from build123d import *

# Parameters (mm, degrees)
CYLINDER009_R     = 5
CYLINDER009_DEPTH = 10
CYLINDER008_R     = 30
CYLINDER008_DEPTH = 10
CYLINDER012_R     = 2
CYLINDER012_DEPTH = 63
CYLINDER013_R     = 2
CYLINDER013_DEPTH = 63
CYLINDER014_R     = 2
CYLINDER014_DEPTH = 63
CYLINDER011_R     = 2
CYLINDER011_DEPTH = 63
BOX004_W          = 86
BOX004_H          = 86
BOX004_DEPTH      = 5
FILLET003_R       = 12
BOX003_W          = 80
BOX003_H          = 80
BOX003_DEPTH      = 1
FILLET002_R       = 12


with BuildPart() as led:
    # Cylinder009 → Cylinder009 (new body)
    with BuildSketch(Plane(origin=(52, 9, -6), x_dir=(1, 0, 0), z_dir=(0, 0, 1))):
        Circle(CYLINDER009_R)
    extrude(amount=CYLINDER009_DEPTH)


with BuildPart() as speaker:
    # Cylinder008 → Cylinder008 (new body)
    with BuildSketch(Plane(origin=(42, 42, -6), x_dir=(1, 0, 0), z_dir=(0, 0, 1))):
        Circle(CYLINDER008_R)
    extrude(amount=CYLINDER008_DEPTH)


with BuildPart() as rod2:
    # Cylinder012 → Cylinder012 (new body)
    with BuildSketch(Plane(origin=(72.6, 72, -9), x_dir=(1, 0, 0), z_dir=(0, 0, 1))):
        Circle(CYLINDER012_R)
    extrude(amount=CYLINDER012_DEPTH)


with BuildPart() as rod3:
    # Cylinder013 → Cylinder013 (new body)
    with BuildSketch(Plane(origin=(12.6, 12, -9), x_dir=(1, 0, 0), z_dir=(0, 0, 1))):
        Circle(CYLINDER013_R)
    extrude(amount=CYLINDER013_DEPTH)


with BuildPart() as rod4:
    # Cylinder014 → Cylinder014 (new body)
    with BuildSketch(Plane(origin=(12.6, 72, -9), x_dir=(1, 0, 0), z_dir=(0, 0, 1))):
        Circle(CYLINDER014_R)
    extrude(amount=CYLINDER014_DEPTH)


with BuildPart() as holes:
    # Cylinder011 → Cylinder011 (new body)
    with BuildSketch(Plane(origin=(72.6, 12, -9), x_dir=(1, 0, 0), z_dir=(0, 0, 1))):
        Circle(CYLINDER011_R)
    extrude(amount=CYLINDER011_DEPTH)

    # Fusion003: union LED, Speaker, rod2, rod3, rod4
    add(led.part)
    add(speaker.part)
    add(rod2.part)
    add(rod3.part)
    add(rod4.part)


with BuildPart() as fillet003:
    # Box004 → Box004 (new body)
    with BuildSketch(Plane.XY):
        with Locations((43, 43)):
            Rectangle(BOX004_W, BOX004_H)
    extrude(amount=BOX004_DEPTH)

    # Fillet003
    fillet003_edges = [fillet003.edges().sort_by_distance(p)[0] for p in [
        (0, 0, 2.5),
        (0, 86, 2.5),
        (86, 0, 2.5),
        (86, 86, 2.5),
    ]]
    fillet(fillet003_edges, radius=FILLET003_R)


with BuildPart() as fillet003_1:
    # Fillet003 placement: moved
    add(fillet003.part.moved(Location((-3, -3, -5))))


with BuildPart() as frontspeaker:
    # Box003 → Box003 (new body)
    with BuildSketch(Plane.XY):
        with Locations((40, 40)):
            Rectangle(BOX003_W, BOX003_H)
    extrude(amount=BOX003_DEPTH)

    # Fillet002
    fillet002_edges = [frontspeaker.edges().sort_by_distance(p)[0] for p in [
        (0, 0, 0.5),
        (0, 80, 0.5),
        (80, 0, 0.5),
        (80, 80, 0.5),
    ]]
    fillet(fillet002_edges, radius=FILLET002_R)

    # Fusion001: union Fillet003
    add(fillet003_1.part)


with BuildPart() as frontspeaker_1:
    # Fusion001 placement: moved
    add(frontspeaker.part.moved(Location((2, 2, 0))))

    # Cut005: cut holes
    add(holes.part, mode=Mode.SUBTRACT)


solid = frontspeaker_1.part
Here's how the part is built. I have some questions about the finished solid (model axes, mm). A direction names the side the tool comes from. Give positions to 0.01 mm unless a question says otherwise; leave off trailing zeros. Order: outer loops, then holes, each group sorted by start corner. A loop starts at its lowest first (then second) coordinate and runs counter-clockwise, first axis right, second up. Notation, with made-up numbers: (41.5, -31) -> (86.5, -31) arc R29 ccw to (86.5, -9) -> close; hole circle Ø4 at (-38.5, 31). An arc over 180 degrees is marked (long way). One line per item, written item: value. Start each with the question number.
1. I need wall thicknesses on probe 1 along Y at (x, z) = (72.6, -1.65); probe 2 along Y at (x, z) = (55.5, -0.3); probe 3 along X at (y, z) = (42, -0.85). Which ranges of each line are inside material? Lowest first, please. Write a range as from..to.
2. For faces 1 (the face through (78.39, 5.42, 0.51)), 2 (the face through (5.42, 78.39, 0.51)), 3 (the face through (39, 1, 0)), 4 (the face through (5.42, 5.61, 0.51)), 5 (the face through (34.543, 71.058, -2.042)), which set-ups out of +Z, -Z, +X, -X, +Y, -Y let a thin tool reach every point of the face, with its end or its side?
3. Imagine slicing it at D-D, the plane z = -2.55. List the corners of the cut face in (x, y) for me, plus the area to 3 significant figures.
4. We'd pull the mould along Y, two halves only. Please class faces 6 (the face through (81.39, 2.42, -2.46)), 7 (the face through (32, 71, -5)), 8 (the face through (78.58, 78.39, 0.51)), 9 (the face through (53.267, 4.163, -2.042)): released by +Y, released by -Y, zero draft, split by the parting line, or undercut.
5. Imagine slicing it at A-A, the plane y = 42. List the corners of the cut face in (x, z) for me, plus the area to 3 significant figures.
6. Imagine slicing it at C-C, the plane x = 56. List the corners of the cut face in (y, z) for me.
7. Will these pins go through, and if not, where does the flat tip stop? pin 1 Ø0.5 at (x, z) = (34.5, 0.5) entering from -Y; pin 2 Ø0.8 at (x, z) = (51, 0.5) entering from +Y.
Values follow:
1. probe 1: y = -1..10, 14..70, 74..85
1. probe 2: y = -1..5.43, 12.57..15.21, 68.79..85
1. probe 3: x = -1..12, 72..85
2. face 1: +Z, +X, -Y
2. face 2: +Z, -X, +Y
2. face 3: +Z
2. face 4: +Z, -X, -Y
2. face 5: +Z, -Z
3. outline: (-1, 11) arc R12 ccw to (11, -1) -> (73, -1) arc R12 ccw to (85, 11) -> (85, 73) arc R12 ccw to (73, 85) -> (11, 85) arc R12 ccw to (-1, 73) -> close; hole circle Ø4 at (12.6, 12); hole circle Ø4 at (12.6, 72); hole (48.7, 12.76) arc R5 ccw (long way) to (52.66, 13.96) arc R30 ccw (long way) to start; hole circle Ø4 at (72.6, 12); hole circle Ø4 at (72.6, 72)
3. area: 4,320 mm2
4. face 6: released by -Y
4. face 7: zero draft
4. face 8: released by +Y
4. face 9: undercut
5. outline: (-1, -5) -> (12, -5) -> (12, 1) -> (2, 1) -> (2, 0) -> (-1, 0) -> close; (72, -5) -> (85, -5) -> (85, 0) -> (82, 0) -> (82, 1) -> (72, 1) -> close
5. area: 150 mm2
6. outline: (-1, -5) -> (6, -5) -> (6, 1) -> (2, 1) -> (2, 0) -> (-1, 0) -> close; (12, -5) -> (15.47, -5) -> (15.47, 1) -> (12, 1) -> close; (68.53, -5) -> (85, -5) -> (85, 0) -> (82, 0) -> (82, 1) -> (68.53, 1) -> close
7. pin 1: stops at y = 2
7. pin 2: stops at y = 82
